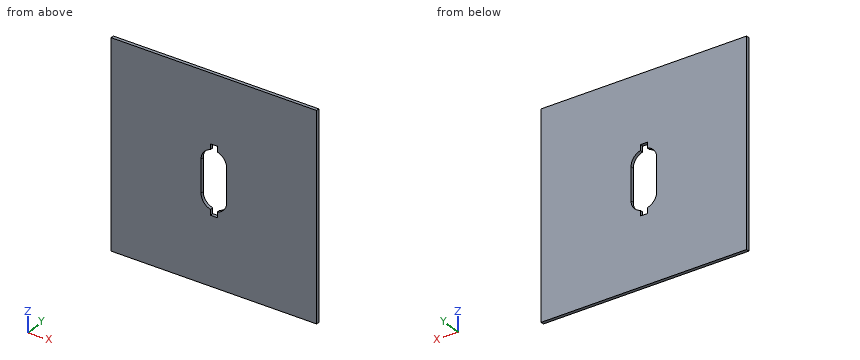
from build123d import *

# Parameters (mm, degrees)
ESQUISSE1_W             = 304.8
ESQUISSE1_H             = 304.8
BOSS_EXTRU_1_DEPTH      = 2.38125
ENL_V_MAT_EXTRU_1_DEPTH = 216.578759172


with BuildPart() as part:
    # Esquisse1 → Boss.-Extru.1 (new, symmetric)
    with BuildSketch(Plane(origin=(0, 0, 0), x_dir=(1, 0, 0), z_dir=(0, 1, 0))):
        Rectangle(ESQUISSE1_W, ESQUISSE1_H)
    extrude(amount=BOSS_EXTRU_1_DEPTH, both=True)

    # Esquisse2 → Enlèv. mat.-Extru.1 (cut, through all)
    with BuildSketch(Plane(origin=(0, 2.38125, 0), x_dir=(1, 0, 0), z_dir=(0, 1, 0))):
        with BuildLine():
            Line((-5.08, -51.10603291), (5.08, -51.10603291))
            Line((5.08, -51.10603291), (5.08, -42.795254256))
            ThreePointArc((5.08, -42.795254256), (15.142330949, -35.978603508), (19.0246, -24.46143291))
            Line((19.0246, -24.46143291), (19.0246, 24.46143291))
            ThreePointArc((19.0246, 24.46143291), (15.142330949, 35.978603508), (5.08, 42.795254256))
            Line((5.08, 42.795254256), (5.08, 50.87496709))
            Line((5.08, 50.87496709), (-5.08, 50.87496709))
            Line((-5.08, 50.87496709), (-5.08, 42.564188437))
            ThreePointArc((-5.08, 42.564188437), (-15.142330949, 35.747537688), (-19.0246, 24.23036709))
            Line((-19.0246, 24.23036709), (-19.0246, -24.46143291))
            ThreePointArc((-19.0246, -24.46143291), (-15.142330949, -35.978603508), (-5.08, -42.795254256))
            Line((-5.08, -42.795254256), (-5.08, -51.10603291))
        make_face()
    extrude(amount=-ENL_V_MAT_EXTRU_1_DEPTH, mode=Mode.SUBTRACT)


solid = part.part
Source: CAD feature listing. Evaluate the final solid. Frame: model axes, mm. Round coordinates to 2 decimals unless told otherwise and drop trailing zeros. Loops run counter-clockwise (first coordinate to the right, second up) from the corner with the lowest first, then second, coordinate; pieces in that order, holes last. Notation, with made-up numbers: (8.25, 76.25) -> (19.25, 76.25) arc R32 cw to (19.25, 109.25) -> close; hole circle Ø5 at (-31.75, 61). An arc over 180 degrees is marked (long way). Answer as a JSON object with one key per item and string values. Group by question number.
Q1. Section query B-B (y = 0.8). Output: boundary loops of the cut face in (x, z), plus the area to 3 significant figures.
Q2. Section query C-C (z = -19). Output: boundary loops of the cut face in (x, y).
Q3. Section query A-A (z = 47). Output: boundary loops of the cut face in (x, y).
Q4. Ray query, line 1 (X direction, y = -0.45, z = 14); line 2 (Z direction, x = -10.5, y = -1.35); line 3 (X direction, y = 2.05, z = 27). Return the intervals inside material, ascending. Write a range as from..to.
Completed:
{
 "1": {"outline": "(-152.4, -152.4) -> (152.4, -152.4) -> (152.4, 152.4) -> (-152.4, 152.4) -> close; hole (-19.02, -24.23) arc R19.02 ccw to (-5.08, -42.56) -> (-5.08, -50.87) -> (5.08, -50.87) -> (5.08, -42.8) arc R19.02 ccw to (19.02, -24.46) -> (19.02, 24.46) arc R19.02 ccw to (5.08, 42.8) -> (5.08, 51.11) -> (-5.08, 51.11) -> (-5.08, 42.8) arc R19.02 ccw to (-19.02, 24.46) -> close", "area": "89,800 mm²"},
 "2": {"outline": "(-152.4, -2.38) -> (-19.02, -2.38) -> (-19.02, 2.38) -> (-152.4, 2.38) -> close; (19.02, -2.38) -> (152.4, -2.38) -> (152.4, 2.38) -> (19.02, 2.38) -> close"},
 "3": {"outline": "(-152.4, -2.38) -> (-5.08, -2.38) -> (-5.08, 2.38) -> (-152.4, 2.38) -> close; (5.08, -2.38) -> (152.4, -2.38) -> (152.4, 2.38) -> (5.08, 2.38) -> close"},
 "4": {"line 1": "-152.4..-19.02, 19.02..152.4", "line 2": "-152.4..-40.09, 40.33..152.4", "line 3": "-152.4..-18.85, 18.85..152.4"}
}
